```python
from build123d import *

# Parameters (mm, degrees)
ESQUISSE1_W             = 12.7
ESQUISSE1_H             = 12.7
BOSS_EXTRU_1_DEPTH      = 29
ESQUISSE2_R             = 2
ENL_V_MAT_EXTRU_1_DEPTH = 13.7
ENL_V_MAT_EXTRU_2_DEPTH = 13.7


with BuildPart() as part:
    # Esquisse1 → Boss.-Extru.1 (new body, symmetric)
    with BuildSketch(Plane.XY):
        Rectangle(ESQUISSE1_W, ESQUISSE1_H)
    extrude(amount=BOSS_EXTRU_1_DEPTH, both=True)

    # Esquisse2 → Enlèv. mat.-Extru.1 (cut, through all)
    with BuildSketch(Plane(origin=(0, 6.35, 0), x_dir=(1, 0, 0), z_dir=(0, 1, 0))):
        with Locations((0, 24.5)):
            Circle(ESQUISSE2_R)
        with Locations((0, 17)):
            Circle(ESQUISSE2_R)
        with Locations((0, -17)):
            Circle(ESQUISSE2_R)
        with Locations((0, -24.5)):
            Circle(ESQUISSE2_R)
    extrude(amount=-ENL_V_MAT_EXTRU_1_DEPTH, mode=Mode.SUBTRACT)

    # Esquisse3 → Enlèv. mat.-Extru.2 (cut, through all)
    with BuildSketch(Plane(origin=(6.35, 0, 0), x_dir=(0, 0, -1), z_dir=(1, 0, 0))):
        with BuildLine():
            ThreePointArc((0, 4.435369207), (-9.15, 0), (0, -4.435369207))
            ThreePointArc((0, -4.435369207), (9.15, 0), (0, 4.435369207))
        make_face()
    extrude(amount=-ENL_V_MAT_EXTRU_2_DEPTH, mode=Mode.SUBTRACT)


solid = part.part
```
Input: part model. Units: mm. Frame: model coordinates. Round coordinates to 2 decimals unless told otherwise and drop trailing zeros. Loops run counter-clockwise (first coordinate to the right, second up) from the corner with the lowest first, then second, coordinate; pieces in that order, holes last. Notation, with made-up numbers: M -20.5,77.25 L 7.5,77.25 A25 cw 7.5,103.25 Z; hole C 21.25,82 d7. An arc over 180 degrees is marked long. Answer in a Markdown table with one row per item. Add a question column.
1. Ray query, probe 1 along Z at (x, y) = (0, 0.25); probe 2 along Z at (x, y) = (-1.75, 5.75); probe 3 along Y at (x, z) = (-3.5, -3.5). Return the intervals inside material, ascending.
2. Section C-C (x = 1.25). Output: boundary loops of the cut face in (y, z), and give its area (3 significant figures).
3. Mould query, pull axis X, two halves, no side actions, for faces 1 (the face through (-6.35, 6, 0)), 2 (the face through (0, 0, -29)), 3 (the face through (0.923, 0.089, 26.274)). Classes: released by +X, released by -X, zero draft, split by the parting line, or undercut.
4. Section A-A (y = 0). Output: boundary loops of the cut face in (x, z), and give its area (3 significant figures).
5. Section D-D (z = 17). Output: boundary loops of the cut face in (x, y), and give its area (3 significant figures).
6. Section B-B (z = 3.5). Output: boundary loops of the cut face in (x, y), and give its area (3 significant figures).
Values follow:
| question | item | result |
|---|---|---|
| 1 | probe 1 | -29 to -26.5, -22.5 to -19, -15 to -9.14, 9.14 to 15, 19 to 22.5, 26.5 to 29 |
| 1 | probe 2 | -29 to -25.47, -23.53 to -17.97, -16.03 to 16.03, 17.97 to 23.53, 25.47 to 29 |
| 1 | probe 3 | -6.35 to -5.65, 5.65 to 6.35 |
| 2 | outline | M -6.35,-29 L 6.35,-29 L 6.35,-26.06 L -6.35,-26.06 Z; M -6.35,-22.94 L 6.35,-22.94 L 6.35,-18.56 L -6.35,-18.56 Z; M -6.35,-15.44 L 6.35,-15.44 L 6.35,15.44 L -6.35,15.44 Z; M -6.35,18.56 L 6.35,18.56 L 6.35,22.94 L -6.35,22.94 Z; M -6.35,26.06 L 6.35,26.06 L 6.35,29 L -6.35,29 Z; hole M -4.44,0 A5.65 ccw long 4.44,0 A5.65 ccw long Z |
| 2 | area | 404 mm^2 |
| 3 | face 1 | released by -X |
| 3 | face 2 | zero draft |
| 3 | face 3 | undercut |
| 4 | outline | M -6.35,-29 L 6.35,-29 L 6.35,-9.15 L -6.35,-9.15 Z; M -6.35,9.15 L 6.35,9.15 L 6.35,29 L -6.35,29 Z; hole C 0,-24.5 d4; hole C 0,-17 d4; hole C 0,17 d4; hole C 0,24.5 d4 |
| 4 | area | 454 mm^2 |
| 5 | outline | M -6.35,-6.35 L -2,-6.35 L -2,6.35 L -6.35,6.35 Z; M 2,-6.35 L 6.35,-6.35 L 6.35,6.35 L 2,6.35 Z |
| 5 | area | 110 mm^2 |
| 6 | outline | M -6.35,-6.35 L 6.35,-6.35 L 6.35,-5.65 L -6.35,-5.65 Z; M -6.35,5.65 L 6.35,5.65 L 6.35,6.35 L -6.35,6.35 Z |
| 6 | area | 17.8 mm^2 |
